Part model, mm, in its own coordinate system. A direction names the side the tool comes from. Round coordinates to 2 decimals unless told otherwise and drop trailing zeros. Loops run counter-clockwise (first coordinate to the right, second up) from the corner with the lowest first, then second, coordinate; pieces in that order, holes last. Notation, with made-up numbers: M 87,39.5 L 124,39.5 A9 cw 124,55.5 Z; hole C 70.25,-13.75 d5. An arc over 180 degrees is marked long. Put each result on its own line as item: value. Start each with the question number.
```python
from build123d import *

# Parameters (mm, degrees)
SKETCH_W        = 60
SKETCH_H        = 65
PAD_DEPTH       = 42
SKETCH001_W     = 50
SKETCH001_H     = 55
POCKET_DEPTH    = 37
SKETCH002_R     = 1.75
POCKET001_DEPTH = 5
SKETCH003_R     = 4
SKETCH003_R_2   = 1.75
PAD001_DEPTH    = 4
SKETCH004_R     = 4.5
POCKET002_DEPTH = 5
SKETCH005_R     = 8.5
POCKET003_DEPTH = 3
POCKET004_DEPTH = 30
POCKET005_DEPTH = 5
PAD002_DEPTH    = 17.5
SKETCH009_R     = 2.75
POCKET006_DEPTH = 36.501
SKETCH010_R     = 4.5
POCKET007_DEPTH = 5
POCKET008_DEPTH = 3
SKETCH012_R     = 1.5
POCKET009_DEPTH = 5


with BuildPart() as part:
    # Sketch → Pad (new body)
    with BuildSketch(Plane.XY):
        Rectangle(SKETCH_W, SKETCH_H)
    extrude(amount=PAD_DEPTH)

    # Sketch001 (on Face6 of Pad) → Pocket (cut)
    with BuildSketch(Plane.XY.offset(42)):
        Rectangle(SKETCH001_W, SKETCH001_H)
    extrude(amount=-POCKET_DEPTH, mode=Mode.SUBTRACT)

    # Sketch002 (on Face4 of Pocket) → Pocket001 (cut)
    with BuildSketch(Plane(origin=(0, 0, 0), x_dir=(1, 0, 0), z_dir=(0, 0, -1))):
        with Locations((-19.5, -22)):
            Circle(SKETCH002_R)
        with Locations((19.5, 22)):
            Circle(SKETCH002_R)
    extrude(amount=-POCKET001_DEPTH, mode=Mode.SUBTRACT)

    # Sketch003 (on Face13 of Pocket001) → Pad001 (join)
    with BuildSketch(Plane.XY.offset(5)):
        with Locations((-19.5, 22)):
            Circle(SKETCH003_R)
        with Locations((-19.5, 22)):
            Circle(SKETCH003_R_2, mode=Mode.SUBTRACT)
        with Locations((19.5, -22)):
            Circle(SKETCH003_R)
        with Locations((19.5, -22)):
            Circle(SKETCH003_R_2, mode=Mode.SUBTRACT)
    extrude(amount=PAD001_DEPTH)

    # Sketch004 (on Face1 of Pad001) → Pocket002 (cut)
    with BuildSketch(Plane(origin=(0, 32.5, 0), x_dir=(-1, 0, 0), z_dir=(0, 1, 0))):
        with Locations((2.5, 23)):
            Circle(SKETCH004_R)
    extrude(amount=-POCKET002_DEPTH, mode=Mode.SUBTRACT)

    # Sketch005 (on Face1 of Pocket002) → Pocket003 (cut)
    with BuildSketch(Plane(origin=(0, 32.5, 0), x_dir=(-1, 0, 0), z_dir=(0, 1, 0))):
        with Locations((2.5, 23)):
            Circle(SKETCH005_R)
    extrude(amount=-POCKET003_DEPTH, mode=Mode.SUBTRACT)

    # Sketch006 (on Face4 of Pocket003) → Pocket004 (cut)
    with BuildSketch(Plane.XY.offset(42)):
        Polygon((-27.5, 28.5), (-26.200962, 30.75), (-28.799038, 30.75), align=None)
        Polygon((27.5, 28.5), (28.799038, 30.75), (26.200962, 30.75), align=None)
        Polygon((28.799038, -30.75), (27.5, -28.5), (26.200962, -30.75), align=None)
        Polygon((-26.200962, -30.75), (-27.5, -28.5), (-28.799038, -30.75), align=None)
    extrude(amount=-POCKET004_DEPTH, mode=Mode.SUBTRACT)

    # Sketch007 (on Face7 of Pocket004) → Pocket005 (cut)
    with BuildSketch(Plane.XZ.offset(32.5)):
        with BuildLine():
            Line((-7.5, 42), (7.5, 42))
            ThreePointArc((2.5, 37), (6.035534, 38.464466), (7.5, 42))
            Line((-2.5, 37), (2.5, 37))
            ThreePointArc((-7.5, 42), (-6.035534, 38.464466), (-2.5, 37))
        make_face()
    extrude(amount=-POCKET005_DEPTH, mode=Mode.SUBTRACT)

    # Sketch008 (on DatumPlane) → Pad002 (join, symmetric)
    with BuildSketch(Plane.XZ):
        with BuildLine():
            Line((-7.5, 0), (7.5, 0))
            Line((7.5, 0), (7.5, -5))
            ThreePointArc((6.5, -31.508887), (14.989339, -18.555827), (7.5, -5))
            Line((6.5, -31.508887), (6.5, -41.508887))
            Line((6.5, -41.508887), (1.5, -41.508887))
            Line((1.5, -41.508887), (1.5, -28.382686))
            ThreePointArc((1.5, -28.382686), (0, -7.490381), (-1.5, -28.382686))
            Line((-1.5, -41.508887), (-1.5, -28.382686))
            Line((-6.5, -41.508887), (-1.5, -41.508887))
            Line((-6.5, -31.508887), (-6.5, -41.508887))
            ThreePointArc((-7.5, -5), (-14.989339, -18.555827), (-6.5, -31.508887))
            Line((-7.5, 0), (-7.5, -5))
        make_face()
    extrude(amount=PAD002_DEPTH, both=True)

    # Sketch009 (on Face36 of Pad002) → Pocket006 (cut, through all)
    with BuildSketch(Plane.YZ.offset(6.5)):
        with Locations((-10.5, -36.508887)):
            Circle(SKETCH009_R)
        with Locations((10.5, -36.508887)):
            Circle(SKETCH009_R)
    extrude(amount=-POCKET006_DEPTH, mode=Mode.SUBTRACT)

    # Sketch010 (on Face1 of Pocket006) → Pocket007 (cut)
    with BuildSketch(Plane(origin=(0, 32.5, 0), x_dir=(-1, 0, 0), z_dir=(0, 1, 0))):
        with Locations((18, 35)):
            Circle(SKETCH010_R)
    extrude(amount=-POCKET007_DEPTH, mode=Mode.SUBTRACT)

    # Sketch011 (on Face1 of Pocket007) → Pocket008 (cut)
    with BuildSketch(Plane(origin=(0, 32.5, 0), x_dir=(-1, 0, 0), z_dir=(0, 1, 0))):
        with BuildLine():
            Line((9, 42), (27, 42))
            Line((27, 42), (27, 32))
            ThreePointArc((9, 32), (18, 26.358899), (27, 32))
            Line((9, 42), (9, 32))
        make_face()
    extrude(amount=-POCKET008_DEPTH, mode=Mode.SUBTRACT)

    # Sketch012 (on Face20 of Pocket008) → Pocket009 (cut)
    with BuildSketch(Plane.XZ.offset(-27.5)):
        with Locations((6, 23)):
            Circle(SKETCH012_R)
    extrude(amount=-POCKET009_DEPTH, mode=Mode.SUBTRACT)


solid = part.part
```
1. Cut at B-B, the plane x = 19.5. Give the cut face in (y, z), and give its area (4 significant figures).
2. Wall check: L1, parallel to Y at x = -19.5, z = 6.45; L2, parallel to Z at x = 6, y = 30; L3, parallel to Z at x = 5.1, y = 10.5. Give the ranges that are in metal, low to high.
3. Which spindle directions (+Z, -Z, +X, -X, +Y, -Y) get a long thin tool onto all of the face, cutting with end or side? Do faces 1 (the flat face through (0, -27.5, 24)), 2 (the flat face through (-6.5, 0, -36)), 3 (the flat face through (-20.1, 29.5, 30.8)), 4 (the flat face through (-10, 17.5, -25)). Say none if no direction does.
4. Mould opens along X. For faces 5 (the cylindrical face through (0.4, -0.2, -7.5)), 6 (the flat face through (21.22, -22.83, 9)), 7 (the cylindrical face through (-15, 0, -18)), 8 (the flat face through (-14, 0, 0)) say: released by +X, released by -X, zero draft, split by the parting line, or undercut.
5. Cut at A-A, the plane z = 35. Give the cut face in (x, y).
6. Drop flat-ended pins along their axis: pin 1 (5.5 mm diameter, centred on x = 19.5, y = -22, fed in from -Z); pin 2 (4 mm diameter, centred on y = 4.5, z = -32.5, fed in from +X); pin 3 (6.5 mm diameter, centred on y = 10.5, z = -36.51, fed in from +X). Give the stop position or say it passes through.
7. Cut at C-C, the plane y = 10.5. Give the cut face in (x, z).
8. Cut at D-D, the plane z = -26. Give the cut face in (x, y).
Results list:
1. outline: M -32.5,0 L -23.75,0 L -23.75,9 L -26,9 L -26,5 L -27.5,5 L -27.5,42 L -32.5,42 Z; M -20.25,0 L 32.5,0 L 32.5,42 L 27.5,42 L 27.5,5 L -18,5 L -18,9 L -20.25,9 Z
1. area: 695.5 mm^2
2. L1: y = -32.5 to -27.5, 18 to 20.25, 23.75 to 26, 27.5 to 32.5
2. L2: z = 0 to 21.5, 24.5 to 42
2. L3: z = -41.51 to -39.26, -33.76 to -27.17, -8.81 to 5
3. face 1: +Z
3. face 2: -Z, -X, +Y, -Y
3. face 3: +Z, +Y
3. face 4: -Z, +X, -X, +Y
4. face 5: undercut
4. face 6: undercut
4. face 7: released by -X
4. face 8: zero draft
5. outline: M -30,-32.5 L 30,-32.5 L 30,32.5 L -9,32.5 L -9,29.5 L -13.5,29.5 L -13.5,27.5 L 25,27.5 L 25,-27.5 L -25,-27.5 L -25,27.5 L -22.5,27.5 L -22.5,29.5 L -26.92,29.5 L -27.5,28.5 L -28.8,30.75 L -27,30.75 L -27,32.5 L -30,32.5 Z; hole M -28.8,-30.75 L -26.2,-30.75 L -27.5,-28.5 Z; hole M 26.2,-30.75 L 28.8,-30.75 L 27.5,-28.5 Z; hole M 26.2,30.75 L 27.5,28.5 L 28.8,30.75 Z
6. pin 1: stops at z = 0
6. pin 2: stops at x = 8.28
6. pin 3: stops at x = 6.5
7. outline: M -30,0 L -7.5,0 L -7.5,-5 A15 ccw -6.5,-31.51 L -6.5,-33.76 L -1.5,-33.76 L -1.5,-28.38 A10.5 cw long 1.5,-28.38 L 1.5,-33.76 L 6.5,-33.76 L 6.5,-31.51 A15 ccw 7.5,-5 L 7.5,0 L 30,0 L 30,42 L 25,42 L 25,5 L -25,5 L -25,42 L -30,42 Z; M -6.5,-41.51 L -1.5,-41.51 L -1.5,-39.26 L -6.5,-39.26 Z; M 1.5,-41.51 L 6.5,-41.51 L 6.5,-39.26 L 1.5,-39.26 Z
8. outline: M -12.68,-17.5 L -6.79,-17.5 L -6.79,17.5 L -12.68,17.5 Z; M 6.79,-17.5 L 12.68,-17.5 L 12.68,17.5 L 6.79,17.5 Z
